```python
from build123d import *

# Parameters (mm, degrees)
SKETCH_1_R      = 2.2
EXTRUDE_1_DEPTH = 5


with BuildPart() as part:
    # 草图1 → 凸台-拉伸1 (new body)
    with BuildSketch(Plane(origin=(0, 0, 0), x_dir=(1, 0, 0), z_dir=(0, 1, 0))):
        Polygon((40, 200), (80, 200), (80, 205), (120, 205), (120, 200), (160, 200), (160, 205), (200, 205), (205, 205), (205, 200), (205, 160), (200, 160), (200, 120), (205, 120), (205, 80), (200, 80), (200, 40), (205, 40), (205, -40), (200, -40), (200, -80), (205, -80), (205, -120), (200, -120), (200, -160), (205, -160), (205, -200), (205, -205), (200, -205), (160, -205), (160, -200), (120, -200), (120, -205), (80, -205), (80, -200), (40, -200), (40, -205), (-40, -205), (-40, -200), (-80, -200), (-80, -205), (-120, -205), (-120, -200), (-160, -200), (-160, -205), (-200, -205), (-205, -205), (-205, -200), (-205, -160), (-200, -160), (-200, -120), (-205, -120), (-205, -80), (-200, -80), (-200, -40), (-205, -40), (-205, 40), (-200, 40), (-200, 80), (-205, 80), (-205, 120), (-200, 120), (-200, 160), (-205, 160), (-205, 200), (-205, 205), (-200, 205), (-160, 205), (-160, 200), (-120, 200), (-120, 205), (-80, 205), (-80, 200), (-40, 200), (-40, 205), (40, 205), align=None)
        with Locations(Location((-190, 0, 0), (0, 0, 270))):
            Circle(SKETCH_1_R, mode=Mode.SUBTRACT)
        with Locations(Location((-190, 40, 0), (0, 0, 270))):
            Circle(SKETCH_1_R, mode=Mode.SUBTRACT)
        with Locations(Location((-190, 80, 0), (0, 0, 270))):
            Circle(SKETCH_1_R, mode=Mode.SUBTRACT)
        with Locations(Location((-190, 120, 0), (0, 0, 270))):
            Circle(SKETCH_1_R, mode=Mode.SUBTRACT)
        with Locations(Location((-190, 160, 0), (0, 0, 270))):
            Circle(SKETCH_1_R, mode=Mode.SUBTRACT)
        with Locations(Location((-190, -160, 0), (0, 0, 270))):
            Circle(SKETCH_1_R, mode=Mode.SUBTRACT)
        with Locations(Location((-190, -120, 0), (0, 0, 270))):
            Circle(SKETCH_1_R, mode=Mode.SUBTRACT)
        with Locations(Location((-190, -80, 0), (0, 0, 270))):
            Circle(SKETCH_1_R, mode=Mode.SUBTRACT)
        with Locations(Location((-190, -40, 0), (0, 0, 270))):
            Circle(SKETCH_1_R, mode=Mode.SUBTRACT)
        with Locations(Location((0, 190, 0), (0, 0, 270))):
            Circle(SKETCH_1_R, mode=Mode.SUBTRACT)
        with Locations(Location((40, 190, 0), (0, 0, 270))):
            Circle(SKETCH_1_R, mode=Mode.SUBTRACT)
        with Locations(Location((80, 190, 0), (0, 0, 270))):
            Circle(SKETCH_1_R, mode=Mode.SUBTRACT)
        with Locations(Location((120, 190, 0), (0, 0, 270))):
            Circle(SKETCH_1_R, mode=Mode.SUBTRACT)
        with Locations(Location((160, 190, 0), (0, 0, 270))):
            Circle(SKETCH_1_R, mode=Mode.SUBTRACT)
        with Locations(Location((-160, 190, 0), (0, 0, 270))):
            Circle(SKETCH_1_R, mode=Mode.SUBTRACT)
        with Locations(Location((-120, 190, 0), (0, 0, 270))):
            Circle(SKETCH_1_R, mode=Mode.SUBTRACT)
        with Locations(Location((-80, 190, 0), (0, 0, 270))):
            Circle(SKETCH_1_R, mode=Mode.SUBTRACT)
        with Locations(Location((-40, 190, 0), (0, 0, 270))):
            Circle(SKETCH_1_R, mode=Mode.SUBTRACT)
        with Locations(Location((190, 0, 0), (0, 0, 270))):
            Circle(SKETCH_1_R, mode=Mode.SUBTRACT)
        with Locations(Location((190, -40, 0), (0, 0, 270))):
            Circle(SKETCH_1_R, mode=Mode.SUBTRACT)
        with Locations(Location((190, -80, 0), (0, 0, 270))):
            Circle(SKETCH_1_R, mode=Mode.SUBTRACT)
        with Locations(Location((190, -120, 0), (0, 0, 270))):
            Circle(SKETCH_1_R, mode=Mode.SUBTRACT)
        with Locations(Location((190, -160, 0), (0, 0, 270))):
            Circle(SKETCH_1_R, mode=Mode.SUBTRACT)
        with Locations(Location((190, 160, 0), (0, 0, 270))):
            Circle(SKETCH_1_R, mode=Mode.SUBTRACT)
        with Locations(Location((190, 120, 0), (0, 0, 270))):
            Circle(SKETCH_1_R, mode=Mode.SUBTRACT)
        with Locations(Location((190, 80, 0), (0, 0, 270))):
            Circle(SKETCH_1_R, mode=Mode.SUBTRACT)
        with Locations(Location((190, 40, 0), (0, 0, 270))):
            Circle(SKETCH_1_R, mode=Mode.SUBTRACT)
        with Locations(Location((0, -190, 0), (0, 0, 270))):
            Circle(SKETCH_1_R, mode=Mode.SUBTRACT)
        with Locations(Location((-40, -190, 0), (0, 0, 270))):
            Circle(SKETCH_1_R, mode=Mode.SUBTRACT)
        with Locations(Location((-80, -190, 0), (0, 0, 270))):
            Circle(SKETCH_1_R, mode=Mode.SUBTRACT)
        with Locations(Location((-120, -190, 0), (0, 0, 270))):
            Circle(SKETCH_1_R, mode=Mode.SUBTRACT)
        with Locations(Location((-160, -190, 0), (0, 0, 270))):
            Circle(SKETCH_1_R, mode=Mode.SUBTRACT)
        with Locations(Location((160, -190, 0), (0, 0, 270))):
            Circle(SKETCH_1_R, mode=Mode.SUBTRACT)
        with Locations(Location((120, -190, 0), (0, 0, 270))):
            Circle(SKETCH_1_R, mode=Mode.SUBTRACT)
        with Locations(Location((80, -190, 0), (0, 0, 270))):
            Circle(SKETCH_1_R, mode=Mode.SUBTRACT)
        with Locations(Location((40, -190, 0), (0, 0, 270))):
            Circle(SKETCH_1_R, mode=Mode.SUBTRACT)
    extrude(amount=EXTRUDE_1_DEPTH)


solid = part.part
```
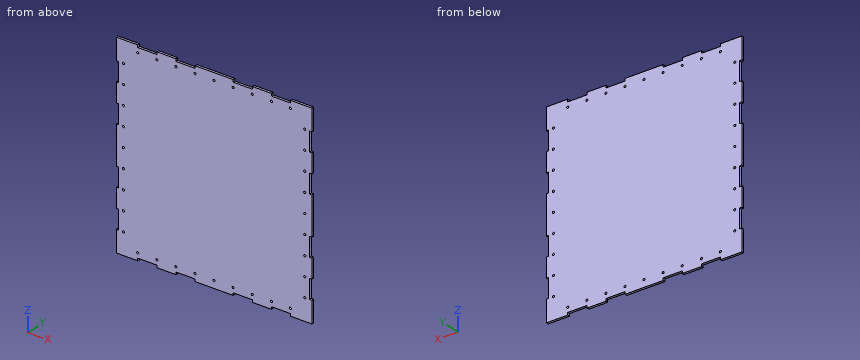
The listing builds one solid part. Answer for the finished solid, in the listing's coordinates (mm). Coordinates: 2 decimals unless noted, no trailing zeros. Order: outer loops, then holes, each group sorted by start corner. A loop starts at its lowest first (then second) coordinate and runs counter-clockwise, first axis right, second up. Notation, with made-up numbers: M 1,-17 L 17,-17 A29 cw 17,8 Z; hole C 56.5,20.5 d10. An arc over 180 degrees is marked long. Answer as a JSON object with one key per item and string values. Group by question number.
1. Section C-C on z = -63.5 is taken. Write down the section's boundary in (x, y), then the cut area to 3 significant figures.
2. Section A-A on y = 1.25 is taken. State how many separate pieces and enclosed holes the cut face has, then the cut area to 3 significant figures.
3. Straight lines are drawn through the part: line 1 (X direction, y = 2.55, z = -79.5); line 2 (X direction, y = 2.1, z = 0); line 3 (Z direction, x = 78, y = 1.75). For each, find the intervals that lie inside material, in ascending order.
4. Section B-B on x = 144.5 is taken. Write down the section's boundary in (y, z).
Values follow:
{
 "1": {"outline": "M -200,0 L 200,0 L 200,5 L -200,5 Z", "area": "2,000 mm2"},
 "2": {"separate pieces": "1", "enclosed holes": "36", "area": "164,000 mm2"},
 "3": {"line 1": "-200 to -192.14, -187.86 to 187.86, 192.14 to 200", "line 2": "-205 to -192.2, -187.8 to 187.8, 192.2 to 205", "line 3": "-200 to -190.92, -189.08 to 189.08, 190.92 to 200"},
 "4": {"outline": "M 0,-200 L 5,-200 L 5,200 L 0,200 Z"}
}
